Can you work these out from the model? Positions are in its coordinate system, mm. A direction names the side the tool comes from. Round coordinates to 2 decimals unless told otherwise and drop trailing zeros. Write each loop counter-clockwise with the first axis right and the second up, starting at its lowest first coordinate (ties: lowest second). Pieces come first, ordered by that corner, then holes. Notation, with made-up numbers: M -21.5,7 L -12.5,7 A26 ccw -12.5,22 Z; hole C 66.5,-37.5 d2. An arc over 180 degrees is marked long. Answer in a Markdown table with one row per item. Add a question column.
(1) Suppose I cut it at B-B, the plane x = -53. Write out the boundary of the cut face in (y, z) (3 decimals).
(2) Suppose I cut it at A-A, the plane z = 13.5. Write out the boundary of the cut face in (x, y) (3 decimals).
(3) If we mould it in two halves opening along Z, with no side actions, what happens to faces 1 (the face through (13, 2, 47.625)), 2 (the face through (16.066, 2, 51)), 3 (the face through (62, 2, 41.529))? For each: released by +Z, released by -Z, zero draft, split by the parting line, or undercut.
(4) For faces 4 (the face through (60.198, 2, 25)), 5 (the face through (-60.198, 2, 25)), 6 (the face through (9.334, 2, 51)), which set-ups out of +Z, -Z, +X, -X, +Y, -Y let a thin tool reach every point of the face, with its end or its side?
(5) I'm going to push flat-ended pins straight in: pin 1 (1.6 mm diameter, centred on y = 2, z = 51, fed in from +X); pin 2 (1 mm diameter, centred on x = -61, y = 2, fed in from -Z); pin 3 (1 mm diameter, centred on x = 38, y = 1.5, fed in from +Z) (3 decimals). Where does each tip first touch, or does it pass through?
(6) If I drill on probe 1 along X at (y, z) = (1.9, 37); probe 2 along Z at (x, y) = (-57, 2.55) (3 decimals), over which ranges is the centre line in solid material (lowest first)?
from build123d import *

# Parameters (mm, degrees)
SKETCH1_W           = 127
SKETCH1_H           = 107.95
BOSS_EXTRUDE1_DEPTH = 3.175
SKETCH2_W           = 3.302
SKETCH2_H           = 6.604
CUT_EXTRUDE1_DEPTH  = 84.400427157
SKETCH3_W           = 127
SKETCH3_H           = 50.8
CUT_EXTRUDE2_DEPTH  = 84.400427157


with BuildPart() as part:
    # Sketch1 → Boss-Extrude1 (new body)
    with BuildSketch(Plane(origin=(0, 0, 0), x_dir=(1, 0, 0), z_dir=(0, 1, 0))):
        Rectangle(SKETCH1_W, SKETCH1_H)
    extrude(amount=BOSS_EXTRUDE1_DEPTH)

    # Sketch2 → Cut-Extrude1 (cut, through all)
    with BuildSketch(Plane.XZ):
        Polygon((-34.7345, 47.625), (-41.4655, 47.625), (-41.4655, 54.229), (-47.4345, 54.229), (-47.4345, 47.625), (-60.198, 47.625), (-63.5, 47.625), (-63.5, 54.229), (-63.5, 63.03162391), (63.5, 63.03162391), (63.5, 54.229), (63.5, 47.625), (60.198, 47.625), (47.4345, 47.625), (47.4345, 54.229), (41.4655, 54.229), (41.4655, 47.625), (34.7345, 47.625), (34.7345, 54.229), (28.7655, 54.229), (28.7655, 47.625), (22.0345, 47.625), (22.0345, 54.229), (16.0655, 54.229), (16.0655, 47.625), (9.3345, 47.625), (9.3345, 54.229), (3.3655, 54.229), (3.3655, 47.625), (-3.3655, 47.625), (-3.3655, 54.229), (-9.3345, 54.229), (-9.3345, 47.625), (-16.0655, 47.625), (-16.0655, 54.229), (-22.0345, 54.229), (-22.0345, 47.625), (-28.7655, 47.625), (-28.7655, 54.229), (-34.7345, 54.229), align=None)
        with Locations((61.849, 38.227)):
            Rectangle(SKETCH2_W, SKETCH2_H)
        with Locations((61.849, 25.527)):
            Rectangle(SKETCH2_W, SKETCH2_H)
        with Locations((61.849, 12.827)):
            Rectangle(SKETCH2_W, SKETCH2_H)
        with Locations((61.849, 0.127)):
            Rectangle(SKETCH2_W, SKETCH2_H)
        with Locations((61.849, -12.573)):
            Rectangle(SKETCH2_W, SKETCH2_H)
        with Locations((61.849, -25.273)):
            Rectangle(SKETCH2_W, SKETCH2_H)
        with Locations((61.849, -37.973)):
            Rectangle(SKETCH2_W, SKETCH2_H)
        with Locations((-61.849, -37.973)):
            Rectangle(SKETCH2_W, SKETCH2_H)
        with Locations((-61.849, -25.273)):
            Rectangle(SKETCH2_W, SKETCH2_H)
        with Locations((-61.849, -12.573)):
            Rectangle(SKETCH2_W, SKETCH2_H)
        with Locations((-61.849, 0.127)):
            Rectangle(SKETCH2_W, SKETCH2_H)
        with Locations((-61.849, 12.827)):
            Rectangle(SKETCH2_W, SKETCH2_H)
        with Locations((-61.849, 25.527)):
            Rectangle(SKETCH2_W, SKETCH2_H)
        with Locations((-61.849, 38.227)):
            Rectangle(SKETCH2_W, SKETCH2_H)
        with Locations((61.849, -50.673)):
            Rectangle(SKETCH2_W, SKETCH2_H)
        with Locations((-61.849, -50.673)):
            Rectangle(SKETCH2_W, SKETCH2_H)
    extrude(amount=-CUT_EXTRUDE1_DEPTH, mode=Mode.SUBTRACT)

    # Sketch3 → Cut-Extrude2 (cut, through all)
    with BuildSketch(Plane(origin=(0, 3.175, 0), x_dir=(1, 0, 0), z_dir=(0, 1, 0))):
        with Locations((0, 28.575)):
            Rectangle(SKETCH3_W, SKETCH3_H)
    extrude(amount=-CUT_EXTRUDE2_DEPTH, mode=Mode.SUBTRACT)


solid = part.part
Calculated:
| question | item | result |
|---|---|---|
| 1 | outline | M 0,-3.175 L 3.175,-3.175 L 3.175,47.625 L 0,47.625 Z |
| 2 | outline | M -60.198,0 L 60.198,0 L 60.198,3.175 L -60.198,3.175 Z |
| 3 | face 1 | released by +Z |
| 3 | face 2 | zero draft |
| 3 | face 3 | undercut |
| 4 | face 4 | +X, +Y, -Y |
| 4 | face 5 | -X, +Y, -Y |
| 4 | face 6 | +Z, +Y, -Y |
| 5 | pin 1 | x = 47.43 |
| 5 | pin 2 | z = 3.43 |
| 5 | pin 3 | z = 47.625 |
| 6 | probe 1 | -60.2 to 60.2 |
| 6 | probe 2 | -3.175 to 47.625 |
